from build123d import *

# Parameters (mm, degrees)
SKETCH1_W           = 431.8
SKETCH1_H           = 330.2
SKETCH1_W_2         = 381
SKETCH1_H_2         = 279.4
BOSS_EXTRUDE1_DEPTH = 6.35
SKETCH2_W           = 25.4
SKETCH2_H           = 25.4
BOSS_EXTRUDE2_DEPTH = 152.4
SKETCH3_W           = 12.7
SKETCH3_H           = 279.4
SKETCH3_W_2         = 381
SKETCH3_H_2         = 12.7
BOSS_EXTRUDE3_DEPTH = 12.7


with BuildPart() as part:
    # Sketch1 → Boss-Extrude1 (new body)
    with BuildSketch(Plane(origin=(0, 0, 0), x_dir=(1, 0, 0), z_dir=(0, 1, 0))):
        Rectangle(SKETCH1_W, SKETCH1_H)
        Rectangle(SKETCH1_W_2, SKETCH1_H_2, mode=Mode.SUBTRACT)
    extrude(amount=BOSS_EXTRUDE1_DEPTH)

    # Sketch2 → Boss-Extrude2 (add)
    with BuildSketch(Plane(origin=(0, 0, 0), x_dir=(1, 0, 0), z_dir=(0, 1, 0))):
        with Locations((-203.2, -152.4)):
            Rectangle(SKETCH2_W, SKETCH2_H)
        with Locations((-203.2, 152.4)):
            Rectangle(SKETCH2_W, SKETCH2_H)
        with Locations((203.2, 152.4)):
            Rectangle(SKETCH2_W, SKETCH2_H)
        with Locations((203.2, -152.4)):
            Rectangle(SKETCH2_W, SKETCH2_H)
    extrude(amount=-BOSS_EXTRUDE2_DEPTH)

    # Sketch3 → Boss-Extrude3 (add)
    with BuildSketch(Plane(origin=(0, 6.35, 0), x_dir=(1, 0, 0), z_dir=(0, 1, 0))):
        with Locations((-209.55, 0)):
            Rectangle(SKETCH3_W, SKETCH3_H)
        with Locations((0, 158.75)):
            Rectangle(SKETCH3_W_2, SKETCH3_H_2)
        with Locations((209.55, 0)):
            Rectangle(SKETCH3_W, SKETCH3_H)
        with Locations((0, -158.75)):
            Rectangle(SKETCH3_W_2, SKETCH3_H_2)
    extrude(amount=BOSS_EXTRUDE3_DEPTH)


solid = part.part
Input: part model. Units: mm. Frame: model coordinates. A direction names the side the tool comes from. Coordinates: 2 decimals unless noted, no trailing zeros. Loops run counter-clockwise (first coordinate to the right, second up) from the corner with the lowest first, then second, coordinate; pieces in that order, holes last.
(1) Section B-B on y = -128.5. Return the cut outline in (x, z).
(2) Material intervals for probe 1 along Z at (x, y) = (41.5, 6.5); probe 2 along X at (y, z) = (-67.5, -146); probe 3 along X at (y, z) = (12, 101), sorted ascending.
(3) Set-up query: faces 1 (the face through (190.5, -75, -152)), 2 (the face through (-3, 13, -152.4)), 3 (the face through (203, -75, -139.7)), 4 (the face through (190.5, 13, 159)). Return all of +Z, -Z, +X, -X, +Y, -Y with unobstructed straight access to the full face (end or side cutting, diameter ignored); none if empty.
(4) First-contact query: pin 1 Ø20.5 at (x, z) = (-201.5, 51.5) entering from -Y; pin 2 Ø4 at (x, y) = (-212.5, 16) entering from -Z. Flat tips, straight axial feed; report the tip coordinate or a pass-through.
(5) Pull-direction query (X, two-part tool) for faces 5 (the face through (-3, 0, -153)), 6 (the face through (215.9, 3, -11)), 7 (the face through (203.2, 13, 2)), 8 (the face through (203, -152.4, 152)); classes: released by +X, released by -X, zero draft, split by the parting line, or undercut.
(6) Section A-A on z = 111. Return the cut outline in (x, y).
(7) Section C-C on x = 185.5. Return the cut outline in (y, z), then the cut area to 3 significant figures.
Data:
1. outline: (-215.9, -165.1) - (-190.5, -165.1) - (-190.5, -139.7) - (-215.9, -139.7) - close; (-215.9, 139.7) - (-190.5, 139.7) - (-190.5, 165.1) - (-215.9, 165.1) - close; (190.5, -165.1) - (215.9, -165.1) - (215.9, -139.7) - (190.5, -139.7) - close; (190.5, 139.7) - (215.9, 139.7) - (215.9, 165.1) - (190.5, 165.1) - close
2. probe 1: z = -165.1 to -152.4, 152.4 to 165.1
2. probe 2: x = -215.9 to -190.5, 190.5 to 215.9
2. probe 3: x = -215.9 to -203.2, 203.2 to 215.9
3. face 1: +Z, -Z, -Y
3. face 2: +X, -X, +Y
3. face 3: +X, -X, -Y
3. face 4: +Z, -Z, +X, +Y
4. pin 1: stops at y = 0
4. pin 2: stops at z = -139.7
5. face 5: undercut
5. face 6: released by +X
5. face 7: undercut
5. face 8: zero draft
6. outline: (-215.9, 0) - (-190.5, 0) - (-190.5, 6.35) - (-203.2, 6.35) - (-203.2, 19.05) - (-215.9, 19.05) - close; (190.5, 0) - (215.9, 0) - (215.9, 19.05) - (203.2, 19.05) - (203.2, 6.35) - (190.5, 6.35) - close
7. outline: (0, -165.1) - (19.05, -165.1) - (19.05, -152.4) - (6.35, -152.4) - (6.35, -139.7) - (0, -139.7) - close; (0, 139.7) - (6.35, 139.7) - (6.35, 152.4) - (19.05, 152.4) - (19.05, 165.1) - (0, 165.1) - close
7. area: 645 mm2
